Source: CAD feature listing. Evaluate the final solid. Frame: model axes, mm. A direction names the side the tool comes from. Give positions to 0.01 mm unless a question says otherwise; leave off trailing zeros. Loops run counter-clockwise (first coordinate to the right, second up) from the corner with the lowest first, then second, coordinate; pieces in that order, holes last. Notation, with made-up numbers: M 75,-10.75 L 120,-10.75 A15 ccw 120,12.25 Z; hole C -14.75,16 d4. An arc over 180 degrees is marked long. Write item = value, one per line.
from build123d import *

# Parameters (mm, degrees)
SKETCH1_W               = 43
SKETCH1_H               = 10
BOSS_EXTRUDE1_DEPTH     = 2
SKETCH2_W               = 3
SKETCH2_H               = 10
BOSS_EXTRUDE2_DEPTH     = 6
SKETCH4_R               = 3.1
BOSS_EXTRUDE3_DEPTH     = 3.6
SKETCH6_R               = 1.7
BOSS_EXTRUDE5_DEPTH     = 1.4
SKETCH7_R               = 2.5
BOSS_EXTRUDE6_DEPTH     = 6
DOME1_FACE_RADIUS       = 2.5
DOME1_HEIGHT            = 2
SKETCH8_R               = 1.15
CUT_EXTRUDE1_DEPTH      = 9
CUT_EXTRUDE1_DEPTH_BACK = 3


with BuildPart() as part:
    # Sketch1 → Boss-Extrude1 (new body)
    with BuildSketch(Plane(origin=(0, 0, 0), x_dir=(1, 0, 0), z_dir=(0, 1, 0))):
        Rectangle(SKETCH1_W, SKETCH1_H)
    extrude(amount=BOSS_EXTRUDE1_DEPTH)

    # Sketch2 → Boss-Extrude2 (add)
    with BuildSketch(Plane(origin=(0, 2, 0), x_dir=(1, 0, 0), z_dir=(0, 1, 0))):
        with Locations((-13, 0.1)):
            Rectangle(SKETCH2_W, SKETCH2_H)
    extrude(amount=BOSS_EXTRUDE2_DEPTH)

    # Sketch4 → Boss-Extrude3 (add)
    with BuildSketch(Plane(origin=(0, 2, 0), x_dir=(1, 0, 0), z_dir=(0, 1, 0))):
        with Locations((-7.4, 0)):
            Circle(SKETCH4_R)
    extrude(amount=BOSS_EXTRUDE3_DEPTH)

    # Sketch6 → Boss-Extrude5 (add)
    with BuildSketch(Plane(origin=(0, 5.6, 0), x_dir=(1, 0, 0), z_dir=(0, 1, 0))):
        with Locations((-7.4, 0)):
            Circle(SKETCH6_R)
    extrude(amount=BOSS_EXTRUDE5_DEPTH)

    # Sketch7 → Boss-Extrude6 (add)
    with BuildSketch(Plane(origin=(0, 2, 0), x_dir=(1, 0, 0), z_dir=(0, 1, 0))):
        with Locations((7.5, 0)):
            Circle(SKETCH7_R)
    extrude(amount=BOSS_EXTRUDE6_DEPTH)

    # Dome1: a dome of height H over a round flat face of radius A is a cap of a sphere of radius (A * A + H * H) / (2 * H)
    dome1_r = (DOME1_FACE_RADIUS * DOME1_FACE_RADIUS + DOME1_HEIGHT * DOME1_HEIGHT) / (2 * DOME1_HEIGHT)
    dome1_base = Plane((7.5, 8, 0), z_dir=(0, 1, 0))
    with Locations(dome1_base.offset(DOME1_HEIGHT - dome1_r)):
        dome1_ball = Sphere(dome1_r, mode=Mode.PRIVATE)
    add(split(dome1_ball, bisect_by=dome1_base, keep=Keep.TOP, mode=Mode.PRIVATE))

    # Sketch8 → Cut-Extrude1 (cut, two sides)
    with BuildSketch(Plane(origin=(0, 2, 0), x_dir=(1, 0, 0), z_dir=(0, 1, 0))) as cut_extrude1_sk:
        with Locations((-18, 0)):
            Circle(SKETCH8_R)
        with Locations((17, 0)):
            Circle(SKETCH8_R)
    extrude(amount=CUT_EXTRUDE1_DEPTH, mode=Mode.SUBTRACT)
    extrude(cut_extrude1_sk.sketch, amount=-CUT_EXTRUDE1_DEPTH_BACK, mode=Mode.SUBTRACT)


solid = part.part
1. Cut plane C-C, the plane z = 3.5. Return the cut outline in (x, y).
Derived:
outline = M -21.5,0 L 21.5,0 L 21.5,2 L -11.5,2 L -11.5,8 L -14.5,8 L -14.5,2 L -21.5,2 Z
2. Pull-direction query (X, two-part tool) for faces 1 (the flat face through (21.5, 1, 0)), 2 (the flat face through (-21.5, 1, 0)), 3 (the flat face through (0, 2, 0)), 4 (the flat face through (-13, 8, 0)); classes: +X half, -X half, draft (parallel to the pull), parting line (faces both ways), or undercut.
Derived:
face_1 = +X half
face_2 = -X half
face_3 = undercut
face_4 = draft
3. First-contact query: pin 1 Ø1 at (x, y) = (1.5, 1.5) entering from -Z; pin 2 Ø1.4 at (x, z) = (-18, 0) entering from +Y; pin 3 Ø1 at (y, z) = (5.5, 1) entering from +X; pin 4 Ø1.5 at (x, z) = (-13, -2.5) entering from +Y. Flat tips, straight axial feed; report the tip coordinate or a pass-through.
Derived:
pin_1 = -5
pin_2 = through
pin_3 = 9.95
pin_4 = 8
4. Reachability of faces 5 (the flat face through (-14.5, 5, 0)), 6 (the flat face through (0, 0, 0)), 7 (the flat face through (-11.5, 5, 0)), 8 (the cylindrical face through (-5.97, 3.77, 2.75)), 9 (the flat face through (-13, 5, 4.9)) from +Z, -Z, +X, -X, +Y, -Y: full face, straight path, thin tool, end or side. Return the list, or none.
Derived:
face_5 = +Z, -Z, -X, +Y
face_6 = +Z, -Z, +X, -X, -Y
face_7 = +Z, -Z, +Y
face_8 = +Y
face_9 = +Z, +X, -X, +Y
5. Cut plane D-D, the plane z = -0.75. Return the cut outline in (x, y), then the cut area to 3 significant figures.
Derived:
outline = M -21.5,0 L -18.87,0 L -18.87,2 L -21.5,2 Z; M -17.13,0 L 16.13,0 L 16.13,2 L 9.88,2 L 9.88,8 A2.45 ccw 5.12,8 L 5.12,2 L -4.39,2 L -4.39,5.6 L -5.87,5.6 L -5.87,7 L -8.93,7 L -8.93,5.6 L -10.41,5.6 L -10.41,2 L -11.5,2 L -11.5,8 L -14.5,8 L -14.5,2 L -17.13,2 Z; M 17.87,0 L 21.5,0 L 21.5,2 L 17.87,2 Z
area = 158 mm²
6. Cut plane A-A, the plane x = -18. Return the cut outline in (y, z), then the cut area to 3 significant figures.
Derived:
outline = M 0,-5 L 2,-5 L 2,-1.15 L 0,-1.15 Z; M 0,1.15 L 2,1.15 L 2,5 L 0,5 Z
area = 15.4 mm²
7. Cut plane B-B, the plane y = 3. Return the cut outline in (x, z).
Derived:
outline = M -14.5,-5.1 L -11.5,-5.1 L -11.5,4.9 L -14.5,4.9 Z; C -7.4,0 d6.2; C 7.5,0 d5
8. Material intervals for probe 1 along X at (y, z) = (1.1, 0); probe 2 along Z at (x, y) = (-18, 1.4); probe 3 along Y at (x, z) = (9, -3), sorted ascending. Write a range as from..to.
Derived:
probe_1 = -21.5..-19.15, -16.85..15.85, 18.15..21.5
probe_2 = -5..-1.15, 1.15..5
probe_3 = 0..2
